```python
from build123d import *

# Parameters (mm, degrees)
BOX043_W                    = 7.5
BOX043_H                    = 27
BOX043_DEPTH                = 4
CYLINDER043_R               = 8.5
CYLINDER043_DEPTH           = 36
BOX042_W                    = 17
BOX042_H                    = 17
BOX042_DEPTH                = 18
BOX039_W                    = 3.4
BOX039_H                    = 24
BOX039_DEPTH                = 100
CYLINDER042_R               = 1.7
CYLINDER042_DEPTH           = 100
CYLINDER042_PLACEMENT_ANGLE = 45
BOX038_W                    = 3.4
BOX038_H                    = 24
BOX038_DEPTH                = 100
CYLINDER041_R               = 1.7
CYLINDER041_DEPTH           = 100
CYLINDER041_PLACEMENT_ANGLE = 45
BOX037_W                    = 3.4
BOX037_H                    = 24
BOX037_DEPTH                = 56
CYLINDER040_R               = 1.7
CYLINDER040_DEPTH           = 56
CYLINDER040_PLACEMENT_ANGLE = 45
BOX041_W                    = 25
BOX041_H                    = 32
BOX041_DEPTH                = 16
BOX041_PLACEMENT_ANGLE      = 45
BOX040_W                    = 22
BOX040_H                    = 17
BOX040_DEPTH                = 16
BOX035_W                    = 41
BOX035_H                    = 17
BOX035_DEPTH                = 122
BOX035_PLACEMENT_ANGLE      = 45
BOX036_W                    = 20
BOX036_H                    = 42
BOX036_DEPTH                = 124
BOX036_PLACEMENT_ANGLE      = 45
BOX034_W                    = 60
BOX034_H                    = 35
BOX034_DEPTH                = 10
BOX033_W                    = 20
BOX033_H                    = 17
BOX033_DEPTH                = 103
FILLET016_R                 = 4


with BuildPart() as cube039:
    # Box043 → Box043 (new body)
    with BuildSketch(Plane(origin=(-3.75, 11, 33), x_dir=(1, 0, 0), z_dir=(0, 0, 1))):
        with Locations((3.75, 13.5)):
            Rectangle(BOX043_W, BOX043_H)
    extrude(amount=BOX043_DEPTH)


with BuildPart() as cylinder015:
    # Cylinder043 → Cylinder043 (new body)
    with BuildSketch(Plane(origin=(0, 10, 121), x_dir=(1, 0, 0), z_dir=(0, 0, 1))):
        Circle(CYLINDER043_R)
    extrude(amount=CYLINDER043_DEPTH)


with BuildPart() as fusion031:
    # Box042 → Box042 (new body)
    with BuildSketch(Plane(origin=(-8.5, -7, 125), x_dir=(1, 0, 0), z_dir=(0, 0, 1))):
        with Locations((8.5, 8.5)):
            Rectangle(BOX042_W, BOX042_H)
    extrude(amount=BOX042_DEPTH)

    # Fusion031: union Cylinder015
    add(cylinder015.part)


with BuildPart() as fusion031_1:
    # Fusion031 placement: moved
    add(fusion031.part.moved(Location((0, -9, 0))))


with BuildPart() as cube035:
    # Box039 → Box039 (new body)
    with BuildSketch(Plane(origin=(20.3, -24, 50), x_dir=(1, 0, 0), z_dir=(0, 0, 1))):
        with Locations((1.7, 12)):
            Rectangle(BOX039_W, BOX039_H)
    extrude(amount=BOX039_DEPTH)


with BuildPart() as fusion029:
    # Cylinder042 → Cylinder042 (new body)
    with BuildSketch(Plane.XY):
        Circle(CYLINDER042_R)
    extrude(amount=CYLINDER042_DEPTH)


with BuildPart() as fusion029_1:
    # Cylinder042 placement: moved
    add(fusion029.part.moved(Location((21.9203, 0, 50))).rotate(Axis((21.9203, 0, 50), (0, 0, 1)), CYLINDER042_PLACEMENT_ANGLE))

    # Fusion029: union Cube035
    add(cube035.part)


with BuildPart() as cube034:
    # Box038 → Box038 (new body)
    with BuildSketch(Plane(origin=(-23.7, -24, 50), x_dir=(1, 0, 0), z_dir=(0, 0, 1))):
        with Locations((1.7, 12)):
            Rectangle(BOX038_W, BOX038_H)
    extrude(amount=BOX038_DEPTH)


with BuildPart() as fusion030:
    # Cylinder041 → Cylinder041 (new body)
    with BuildSketch(Plane.XY):
        Circle(CYLINDER041_R)
    extrude(amount=CYLINDER041_DEPTH)


with BuildPart() as fusion030_1:
    # Cylinder041 placement: moved
    add(fusion030.part.moved(Location((-21.9203, 0, 50))).rotate(Axis((-21.9203, 0, 50), (0, 0, 1)), CYLINDER041_PLACEMENT_ANGLE))

    # Fusion030: union Cube034
    add(cube034.part)


with BuildPart() as cube033:
    # Box037 → Box037 (new body)
    with BuildSketch(Plane(origin=(-1.7, -2, -3), x_dir=(1, 0, 0), z_dir=(0, 0, 1))):
        with Locations((1.7, 12)):
            Rectangle(BOX037_W, BOX037_H)
    extrude(amount=BOX037_DEPTH)


with BuildPart() as top_slot:
    # Cylinder040 → Cylinder040 (new body)
    with BuildSketch(Plane.XY):
        Circle(CYLINDER040_R)
    extrude(amount=CYLINDER040_DEPTH)


with BuildPart() as top_slot_1:
    # Cylinder040 placement: moved
    add(top_slot.part.moved(Location((0, 21.92031, -3))).rotate(Axis((0, 21.92031, -3), (0, 0, 1)), CYLINDER040_PLACEMENT_ANGLE))

    # Fusion028: union Cube033
    add(cube033.part)


with BuildPart() as top_slot_2:
    # Fusion028 placement: moved
    add(top_slot_1.part.moved(Location((0, 0, -6))))


with BuildPart() as cube037:
    # Box041 → Box041 (new body)
    with BuildSketch(Plane.XY):
        with Locations((12.5, 16)):
            Rectangle(BOX041_W, BOX041_H)
    extrude(amount=BOX041_DEPTH)


with BuildPart() as cube037_1:
    # Box041 placement: moved
    add(cube037.part.moved(Location((-13, 18, 35))).rotate(Axis((-13, 18, 35), (1, 0, 0)), BOX041_PLACEMENT_ANGLE))


with BuildPart() as cut052:
    # Box040 → Box040 (new body)
    with BuildSketch(Plane(origin=(-11, 18, 33), x_dir=(1, 0, 0), z_dir=(0, 0, 1))):
        with Locations((11, 8.5)):
            Rectangle(BOX040_W, BOX040_H)
    extrude(amount=BOX040_DEPTH)

    # Cut052: cut Cube037
    add(cube037_1.part, mode=Mode.SUBTRACT)


with BuildPart() as cube031:
    # Box035 → Box035 (new body)
    with BuildSketch(Plane.XY):
        with Locations((20.5, 8.5)):
            Rectangle(BOX035_W, BOX035_H)
    extrude(amount=BOX035_DEPTH)


with BuildPart() as cube031_1:
    # Box035 placement: moved
    add(cube031.part.moved(Location((-31, 5, 19))).rotate(Axis((-31, 5, 19), (0, 0, 1)), BOX035_PLACEMENT_ANGLE))


with BuildPart() as cube032:
    # Box036 → Box036 (new body)
    with BuildSketch(Plane.XY):
        with Locations((10, 21)):
            Rectangle(BOX036_W, BOX036_H)
    extrude(amount=BOX036_DEPTH)


with BuildPart() as cube032_1:
    # Box036 placement: moved
    add(cube032.part.moved(Location((33, 3, 19))).rotate(Axis((33, 3, 19), (0, 0, 1)), BOX036_PLACEMENT_ANGLE))


with BuildPart() as cube030:
    # Box034 → Box034 (new body)
    with BuildSketch(Plane(origin=(-30, -5, 126), x_dir=(1, 0, 0), z_dir=(0, 0, 1))):
        with Locations((30, 17.5)):
            Rectangle(BOX034_W, BOX034_H)
    extrude(amount=BOX034_DEPTH)


with BuildPart() as obj1:
    # Box033 → Box033 (new body)
    with BuildSketch(Plane(origin=(-10, 13, 23), x_dir=(1, 0, 0), z_dir=(0, 0, 1))):
        with Locations((10, 8.5)):
            Rectangle(BOX033_W, BOX033_H)
    extrude(amount=BOX033_DEPTH)

    # Fusion027: union Cube030
    add(cube030.part)

    # Cut050: cut Cube032
    add(cube032_1.part, mode=Mode.SUBTRACT)

    # Cut051: cut Cube031
    add(cube031_1.part, mode=Mode.SUBTRACT)

    # Cut053: cut Cut052
    add(cut052.part, mode=Mode.SUBTRACT)

    # Cut054: cut top-slot
    add(top_slot_2.part, mode=Mode.SUBTRACT)

    # Cut055: cut Fusion030
    add(fusion030_1.part, mode=Mode.SUBTRACT)

    # Cut056: cut Fusion029
    add(fusion029_1.part, mode=Mode.SUBTRACT)

    # Cut057: cut Fusion031
    add(fusion031_1.part, mode=Mode.SUBTRACT)

    # Cut058: cut Cube039
    add(cube039.part, mode=Mode.SUBTRACT)

    # Fillet016
    fillet016_edges = [obj1.edges().sort_by_distance(p)[0] for p in [
        (0, 13, 126),
    ]]
    fillet(fillet016_edges, radius=FILLET016_R)


solid = obj1.part
```
The listing builds one solid part. Answer for the finished solid, in the listing's coordinates (mm). A direction names the side the tool comes from. Coordinates: 2 decimals unless noted, no trailing zeros. Loops run counter-clockwise (first coordinate to the right, second up) from the corner with the lowest first, then second, coordinate; pieces in that order, holes last. Notation, with made-up numbers: (-28.5, 87) - (29.5, 87) arc R19 cw to (29.5, 113) - close; hole circle Ø3 at (46, -23.5). An arc over 180 degrees is marked (long way). Write item = value, one per line.
1) Each of these flat-tipped pins is pushed along its axis until it touches: P1, Ø10, axis at x = 3.5, z = 71.5, coming from the -Y side; P2, Ø8, axis at x = 17.5, y = 16.5, coming from the -Z side; P3, Ø1.7, axis at x = 0.5, y = 18.5, coming from the -Z side; P4, Ø2, axis at x = 21.92, y = 0, coming from the -Z side. Where does it stop, or does it pass through?
Responses:
P1 = 13
P2 = 126
P3 = 47
P4 = through
2) Section B-B (x = 12) is taken. Determine the outline of the cut face in (y, z), plus the area to 3 significant figures.
Responses:
outline = (-5, 126) - (24, 126) - (24, 136) - (-5, 136) - close
area = 290 mm^2
3) Which of the six approach directions +Z, -Z, +X, -X, +Y, -Y give full straight-line access (tool end or side, diameter ignored) to faces 4 (the face through (23.7, -3, 131)), 5 (the face through (7, 18, 34)), 6 (the face through (1.7, 17, 28)), 7 (the face through (0, 13, 72))?
Responses:
face_4 = +Z, -Z, -Y
face_5 = +X, -X, +Y
face_6 = -Z, -Y
face_7 = -Z, +X, -X, -Y
4) Find the intervals of material crossed by line 1 along Y through (x, z) = (1, 112); line 2 along Z through (x, y) = (17, 12); line 3 along X through (y, z) = (22, 62), in increasing order.
Responses:
line_1 = 13 to 30
line_2 = 126 to 136
line_3 = -10 to 10
5) Section C-C (z = 101) is taken. Determine the outline of the cut face in (x, y).
Responses:
outline = (-10, 13) - (10, 13) - (10, 26) - (6, 30) - (-6, 30) - (-10, 26) - close
6) Determine the mould class of faces 1 (the face through (1.7, 17, 42)), 2 (the face through (-8, 28, 28)), 3 (the face through (-2, 22, 23)) for opening direction X: pulls with the +X half, pulls with the -X half, needs draft (parallel to the pull), parting line crosses it, or undercut.
Responses:
face_1 = undercut
face_2 = pulls with the -X half
face_3 = needs draft
7) Section D-D (x = -17) is taken. Determine the outline of the cut face in (y, z), plus the area to 3 significant figures.
Responses:
outline = (-5, 126) - (19, 126) - (19, 136) - (-5, 136) - close
area = 240 mm^2
